```python
from build123d import *

# Parameters (mm, degrees)
BOSS_EXTRUDE1_DEPTH = 14
SKETCH3_W           = 20
SKETCH3_H           = 20
BOSS_EXTRUDE2_DEPTH = 30
SKETCH4_W           = 18
SKETCH4_H           = 18
CUT_EXTRUDE1_DEPTH  = 3
FILLET2_R           = 2
FILLET3_R           = 2
CUT_EXTRUDE2_DEPTH  = 0.5
BOSS_EXTRUDE3_DEPTH = 0.2
SKETCH8_W           = 10
SKETCH8_H           = 4
CUT_EXTRUDE4_DEPTH  = 20


with BuildPart() as part:
    # Sketch1 → Boss-Extrude1 (new body)
    with BuildSketch(Plane(origin=(0, 0, 0), x_dir=(1, 0, 0), z_dir=(0, 1, 0))):
        with BuildLine():
            Line((0, 5), (10, 5))
            Line((10, 5), (10, -5))
            Line((10, -5), (0, -5))
            ThreePointArc((0, -5), (-5, 0), (0, 5))
        make_face()
    extrude(amount=BOSS_EXTRUDE1_DEPTH)

    # Sketch3 → Boss-Extrude2 (add)
    with BuildSketch(Plane(origin=(10, 0, 0), x_dir=(0, 0, -1), z_dir=(1, 0, 0))):
        with Locations((0, 7)):
            Rectangle(SKETCH3_W, SKETCH3_H)
    extrude(amount=BOSS_EXTRUDE2_DEPTH)

    # Sketch4 → Cut-Extrude1 (cut)
    with BuildSketch(Plane(origin=(40, 0, 0), x_dir=(0, 0, -1), z_dir=(1, 0, 0))):
        with Locations((0, 7)):
            Rectangle(SKETCH4_W, SKETCH4_H)
    extrude(amount=-CUT_EXTRUDE1_DEPTH, mode=Mode.SUBTRACT)

    # Fillet2
    fillet2_edges = [part.edges().sort_by_distance(p)[0] for p in [
        (25, -3, -10),
        (25, 17, -10),
        (25, 17, 10),
        (25, -3, 10),
    ]]
    fillet(fillet2_edges, radius=FILLET2_R)

    # Fillet3
    fillet3_edges = [part.edges().sort_by_distance(p)[0] for p in [
        (38.5, 16, -9),
        (38.5, -2, -9),
        (38.5, -2, 9),
        (38.5, 16, 9),
    ]]
    fillet(fillet3_edges, radius=FILLET3_R)

    # Sketch5 → Cut-Extrude2 (cut)
    with BuildSketch(Plane(origin=(37, 0, 0), x_dir=(0, 0, -1), z_dir=(1, 0, 0))):
        with BuildLine():
            ThreePointArc((4, 7), (1.530733729, 10.69551813), (-2.828427125, 9.828427125))
            Line((-2.828427125, 9.828427125), (2.828427125, 4.171572875))
            ThreePointArc((2.828427125, 4.171572875), (3.69551813, 5.469266271), (4, 7))
        make_face()
        with BuildLine():
            Line((2.828427125, 4.171572875), (-2.828427125, 9.828427125))
            ThreePointArc((-2.828427125, 9.828427125), (-2.828427125, 4.171572875), (2.828427125, 4.171572875))
        make_face()
    extrude(amount=-CUT_EXTRUDE2_DEPTH, mode=Mode.SUBTRACT)

    # Sketch6 → Boss-Extrude3 (add)
    with BuildSketch(Plane(origin=(39, 0, 0), x_dir=(0, 0, -1), z_dir=(1, 0, 0))):
        with BuildLine():
            Line((-7, 16), (7, 16))
            ThreePointArc((7, 16), (8.414213562, 15.414213562), (9, 14))
            Line((9, 14), (9, 0))
            ThreePointArc((9, 0), (8.414213562, -1.414213562), (7, -2))
            Line((7, -2), (-7, -2))
            ThreePointArc((-7, -2), (-8.414213562, -1.414213562), (-9, 0))
            Line((-9, 0), (-9, 14))
            ThreePointArc((-9, 14), (-8.414213562, 15.414213562), (-7, 16))
        make_face()
    extrude(amount=BOSS_EXTRUDE3_DEPTH)

    # Sketch8 → Cut-Extrude4 (cut)
    with BuildSketch(Plane(origin=(0, 0, -5), x_dir=(-1, 0, 0), z_dir=(0, 0, -1))):
        with Locations((0, 7)):
            Rectangle(SKETCH8_W, SKETCH8_H)
    extrude(amount=-CUT_EXTRUDE4_DEPTH, mode=Mode.SUBTRACT)


solid = part.part
```
CAD build for the part. Positions are in the model's coordinates, mm. A direction names the side the tool comes from. Give positions to 0.01 mm unless a question says otherwise; leave off trailing zeros. Order: outer loops, then holes, each group sorted by start corner. A loop starts at its lowest first (then second) coordinate and runs counter-clockwise, first axis right, second up.
(1) Saw through at A-A, the plane z = 0. Give the cut face in (x, y).
(2) Saw through at D-D, the plane z = -5.75. Give the cut face in (x, y), then the cut area to 3 significant figures.
(3) Drill centre lines: L1, parallel to X at y = 14, z = 8.25; L2, parallel to Y at x = 38, z = 3; L3, parallel to Y at x = 9, z = -0.5. Where is each one in solid material? Low to high.
(4) Tool access for faces 1 (the flat face through (6, 7, 5)), 2 (the cylindrical face through (39.59, -1.43, 8.4)), 3 (the flat face through (3, 14, 0)), 4 (the cylindrical face through (37.99, 15.43, 8.4)): list every direction of +Z, -Z, +X, -X, +Y, -Y with a clear straight run to the whole face (end or side of a thin tool).
(5) Flat gauge pins, fed straight in: pin 1 (5 mm diameter, centred on x = 6, y = 10, fed in from +Z); pin 2 (11 mm diameter, centred on x = 1, z = -0.5, fed in from +Y); pin 3 (4 mm diameter, centred on y = 2.5, z = 5.5, fed in from -X). Where does each tip first touch, or does it go through?
(6) Saw through at B-B, the plane x = -2. Give the cut face in (y, z), then the cut area to 3 significant figures.
(7) Saw through at C-C, the plane x = 9.5. Give the cut face in (y, z).
(8) Mould opens along Z. For faces 5 (the flat face through (0, 9, 0)), 6 (the flat face through (25, 7, -10)), 7 (the flat face through (36.5, 7, 0)) say: released by +Z, released by -Z, zero draft, split by the parting line, or undercut.
Results found:
1. outline: (-5, 0) - (10, 0) - (10, -3) - (40, -3) - (40, -2) - (39.2, -2) - (39.2, 16) - (40, 16) - (40, 17) - (10, 17) - (10, 14) - (-5, 14) - (-5, 9) - (5, 9) - (5, 5) - (-5, 5) - close; hole (36.5, 3) - (37, 3) - (37, -2) - (39, -2) - (39, 16) - (37, 16) - (37, 11) - (36.5, 11) - close
2. outline: (10, -3) - (40, -3) - (40, -2) - (39.2, -2) - (39.2, 16) - (40, 16) - (40, 17) - (10, 17) - close; hole (37, -2) - (39, -2) - (39, 16) - (37, 16) - close
2. area: 550 mm2
3. L1: x = 10 to 37, 39 to 39.2
3. L2: y = -3 to -2, 16 to 17
3. L3: y = 0 to 14
4. face 1: +Z, -X, +Y, -Y
4. face 2: +X
4. face 3: +Z, -Z, -X, +Y
4. face 4: none
5. pin 1: stops at z = 5
5. pin 2: stops at y = 14
5. pin 3: stops at x = -3.57
6. outline: (0, -4.58) - (5, -4.58) - (5, 4.58) - (0, 4.58) - close; (9, -4.58) - (14, -4.58) - (14, 4.58) - (9, 4.58) - close
6. area: 91.7 mm2
7. outline: (0, -5) - (14, -5) - (14, 5) - (0, 5) - close
8. face 5: zero draft
8. face 6: released by -Z
8. face 7: undercut
